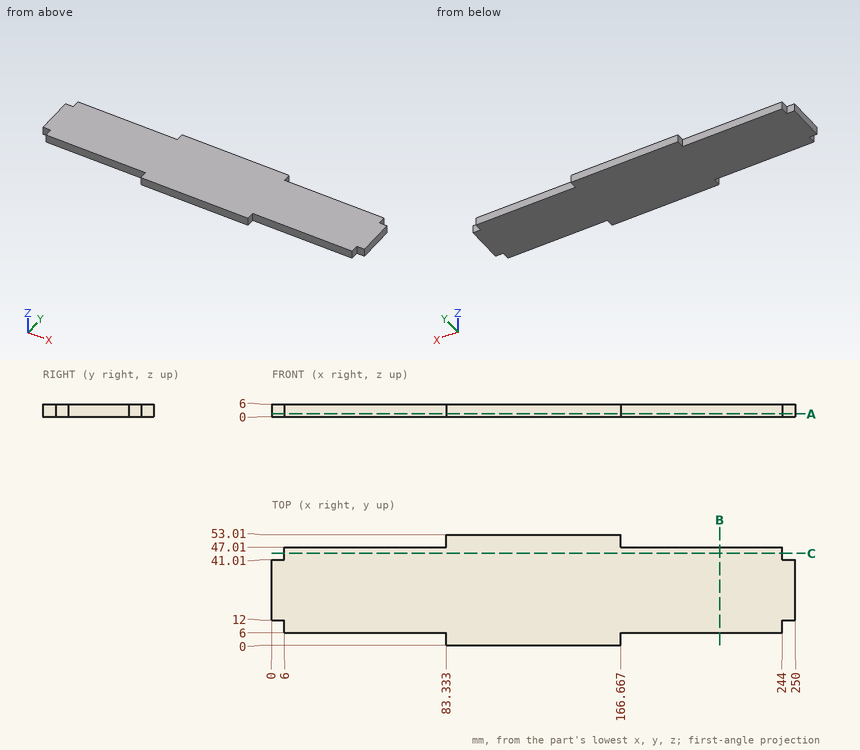
Verification items for this drawing (mm, ordinates from the low corner). Coordinates: 2 decimals unless noted, no trailing zeros. Order: outer loops, then holes, each group sorted by start corner. A loop starts at its lowest first (then second) coordinate and runs counter-clockwise, first axis right, second up. Notation, with made-up numbers: (-28, -30.5) -> (20, -30.5) arc R11 cw to (20, -17.5) -> close; hole circle Ø8 at (71.25, 16). An arc over 180 degrees is marked (long way). Put each result on its own line as item: value. Start each with the question number.
1. Cross-section at C-C, the plane y = 44. Record the boundary of the cut face in (x, z).
2. Cross-section at B-B, the plane x = 214. Record the boundary of the cut face in (y, z).
3. Go/stop test with flat-tipped pins: pin 1 Ø3 at (x, z) = (3.5, 3) entering from +Y; pin 2 Ø1.8 at (x, z) = (29, 2.5) entering from +Y; pin 3 Ø5 at (x, y) = (163.5, 29.5) entering from -Z; pin 4 Ø1.8 at (y, z) = (3.5, 3.5) entering from -X. Record where each tip stops, or that it passes through.
4. Material ranges on L1, parallel to Y at x = 201, z = 3.65; L2, parallel to X at y = 49, z = 4.5; L3, parallel to X at y = 11.5, z = 2.15, recorded low to high. Write a range as [from, to].
5. Cross-section at A-A, the plane z = 1.25. Record the boundary of the cut face in (x, y).
Computed:
1. outline: (6, 0) -> (244, 0) -> (244, 6) -> (6, 6) -> close
2. outline: (6, 0) -> (47.01, 0) -> (47.01, 6) -> (6, 6) -> close
3. pin 1: y = 41.01
3. pin 2: y = 47.01
3. pin 3: z = 0
3. pin 4: x = 83.33
4. L1: [6, 47.01]
4. L2: [83.33, 166.67]
4. L3: [6, 244]
5. outline: (0, 12) -> (6, 12) -> (6, 6) -> (83.33, 6) -> (83.33, 0) -> (166.67, 0) -> (166.67, 6) -> (244, 6) -> (244, 12) -> (250, 12) -> (250, 41.01) -> (244, 41.01) -> (244, 47.01) -> (166.67, 47.01) -> (166.67, 53.01) -> (83.33, 53.01) -> (83.33, 47.01) -> (6, 47.01) -> (6, 41.01) -> (0, 41.01) -> close
